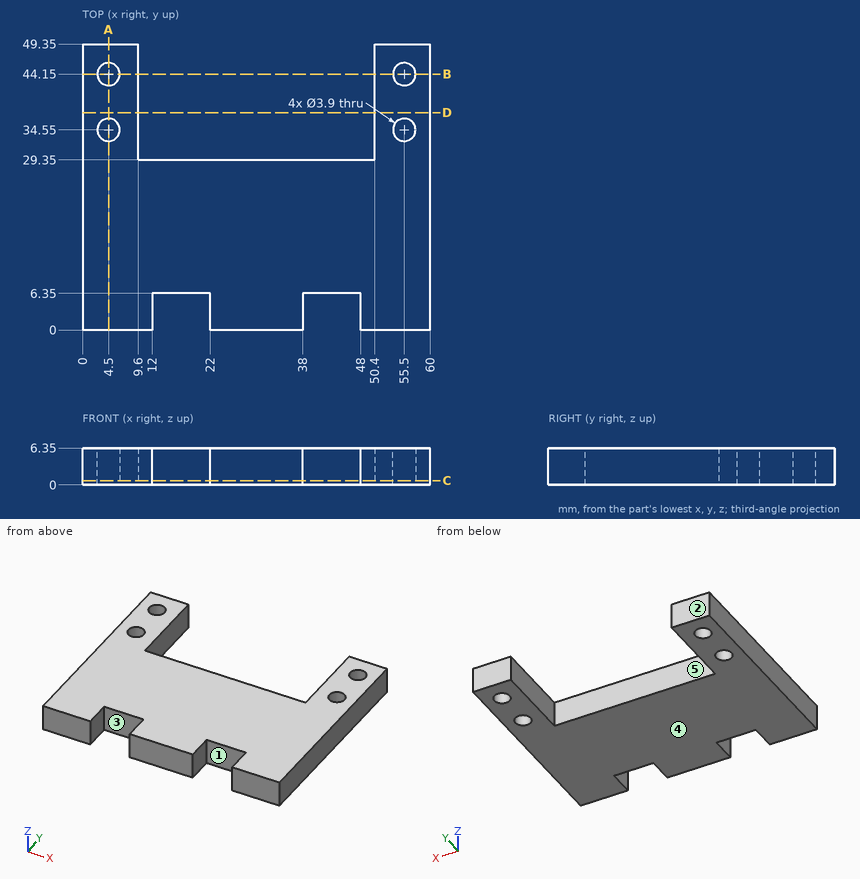
Geometry check sheet. Reference: drawing and pictorial views, mm from the part's lowest x, y, z. A direction names the side the tool comes from. Give positions to 0.01 mm unless a question says otherwise; leave off trailing zeros. Write each loop counter-clockwise with the first axis right and the second up, starting at its lowest first coordinate (ties: lowest second). Pieces come first, ordered by that corner, then holes.
Item 1: Cross-section at A-A (x = 4.5). Enter the section's corners in (y, z), and give its area (3 significant figures).
Item 2: Cross-section at B-B (y = 44.15). Enter the section's corners in (x, z).
Item 3: Draft check along X on the marked faces 1 and 2. Enter one of: released by +X, released by -X, zero draft, split by the parting line, or undercut.
Item 4: Cross-section at D-D (y = 37.5). Enter the section's corners in (x, z), and give its area (3 significant figures).
Item 5: Scan lines: L1, parallel to Y at x = 4.5, z = 4.75; L2, parallel to X at y = 33.5, z = 3.5; L3, parallel to Y at x = 13, z = 3.25. Record each from-to range of solid material in increasing order.
Item 6: Gauge pin test, flat ends, axial feed: pin 1 (3 mm diameter, centred on y = 3.5, z = 4.5, fed in from -X); pin 2 (3 mm diameter, centred on x = 21.5, z = 4.5, fed in from +Y); pin 3 (2 mm diameter, centred on x = 20, z = 4, fed in from -Y). Record the tip position at first contact, or that the pin passes through.
Item 7: Cross-section at C-C (z = 0.75). Enter the section's corners in (x, y).
Item 8: Access from +Z, -Z, +X, -X, +Y, -Y to the whole of each face (thin tool, end or side, straight path). Record for the marked faces 3, 4 and 5.
Report:
1. outline: (0, 0) - (32.6, 0) - (32.6, 6.35) - (0, 6.35) - close; (36.5, 0) - (42.2, 0) - (42.2, 6.35) - (36.5, 6.35) - close; (46.1, 0) - (49.35, 0) - (49.35, 6.35) - (46.1, 6.35) - close
1. area: 264 mm2
2. outline: (0, 0) - (2.55, 0) - (2.55, 6.35) - (0, 6.35) - close; (6.45, 0) - (9.6, 0) - (9.6, 6.35) - (6.45, 6.35) - close; (50.4, 0) - (53.55, 0) - (53.55, 6.35) - (50.4, 6.35) - close; (57.45, 0) - (60, 0) - (60, 6.35) - (57.45, 6.35) - close
3. face 1: undercut
3. face 2: zero draft
4. outline: (0, 0) - (9.6, 0) - (9.6, 6.35) - (0, 6.35) - close; (50.4, 0) - (60, 0) - (60, 6.35) - (50.4, 6.35) - close
4. area: 122 mm2
5. L1: y = 0 to 32.6, 36.5 to 42.2, 46.1 to 49.35
5. L2: x = 0 to 2.86, 6.14 to 9.6, 50.4 to 53.86, 57.14 to 60
5. L3: y = 6.35 to 29.35
6. pin 1: stops at x = 0
6. pin 2: stops at y = 29.35
6. pin 3: stops at y = 6.35
7. outline: (0, 0) - (12, 0) - (12, 6.35) - (22, 6.35) - (22, 0) - (38, 0) - (38, 6.35) - (48, 6.35) - (48, 0) - (60, 0) - (60, 49.35) - (50.4, 49.35) - (50.4, 29.35) - (9.6, 29.35) - (9.6, 49.35) - (0, 49.35) - close; hole circle Ø3.9 at (4.5, 34.55); hole circle Ø3.9 at (4.5, 44.15); hole circle Ø3.9 at (55.5, 34.55); hole circle Ø3.9 at (55.5, 44.15)
8. face 3: +Z, -Z, -Y
8. face 4: -Z, +X, -X, +Y, -Y
8. face 5: +Z, -Z, +Y
